from build123d import *

# Parameters (mm, degrees)
BOSS_EXTRUDE1_DEPTH = 8
CUT_EXTRUDE1_DEPTH  = 90
SKETCH3_R           = 5
CUT_EXTRUDE2_DEPTH  = 5.4
SKETCH5_R           = 2.2
SKETCH5_R_2         = 4.65
CUT_EXTRUDE3_DEPTH  = 20
SKETCH6_R           = 20.6
SKETCH6_R_2         = 15.6
CUT_EXTRUDE4_DEPTH  = 2.5
SKETCH7_R           = 20.6
SKETCH7_R_2         = 15.6
CUT_EXTRUDE5_DEPTH  = 2.5
CUT_EXTRUDE6_REACH  = 127.974
SKETCH9_R           = 2.2
SKETCH9_R_2         = 6.575


with BuildPart() as part:
    # Sketch1 → Boss-Extrude1 (new body)
    with BuildSketch(Plane.XY):
        with BuildLine():
            Line((-83.790627288, -89.5), (83.790627288, -89.5))
            ThreePointArc((83.790627288, -89.5), (86.972607803, -88.181980515), (88.290627288, -85))
            Line((88.290627288, -85), (88.290627288, 85))
            ThreePointArc((88.290627288, 85), (86.972607803, 88.181980515), (83.790627288, 89.5))
            Line((83.790627288, 89.5), (-83.790627288, 89.5))
            ThreePointArc((-83.790627288, 89.5), (-86.972607803, 88.181980515), (-88.290627288, 85))
            Line((-88.290627288, 85), (-88.290627288, -85))
            ThreePointArc((-88.290627288, -85), (-86.972607803, -88.181980515), (-83.790627288, -89.5))
        make_face()
    extrude(amount=BOSS_EXTRUDE1_DEPTH)

    # Sketch2 → Cut-Extrude1 (cut)
    with BuildSketch(Plane.XY.offset(8)):
        with BuildLine():
            ThreePointArc((43.745313644, 83.5), (41.145313644, 86.1), (38.545313644, 83.5))
            ThreePointArc((38.545313644, 83.5), (41.145313644, 80.9), (43.745313644, 83.5))
        make_face()
        with BuildLine():
            Line((0, 84), (2.551470164, 84))
            ThreePointArc((2.551470164, 84), (0, 86.1), (-2.551470164, 84))
            Line((-2.551470164, 84), (0, 84))
        make_face()
        with BuildLine():
            Line((0, 84), (-2.551470164, 84))
            ThreePointArc((-2.551470164, 84), (0, 80.9), (2.551470164, 84))
            Line((2.551470164, 84), (0, 84))
        make_face()
        with BuildLine():
            ThreePointArc((-43.745313644, 83.5), (-41.145313644, 80.9), (-38.545313644, 83.5))
            ThreePointArc((-38.545313644, 83.5), (-41.145313644, 86.1), (-43.745313644, 83.5))
        make_face()
        with BuildLine():
            ThreePointArc((-84.890627288, 83.5), (-82.290627288, 80.9), (-79.690627288, 83.5))
            ThreePointArc((-79.690627288, 83.5), (-82.290627288, 86.1), (-84.890627288, 83.5))
        make_face()
        with BuildLine():
            ThreePointArc((-84.890627288, 41.75), (-82.290627288, 39.15), (-79.690627288, 41.75))
            ThreePointArc((-79.690627288, 41.75), (-82.290627288, 44.35), (-84.890627288, 41.75))
        make_face()
        with BuildLine():
            ThreePointArc((-84.890627288, 0), (-82.290627288, -2.6), (-79.690627288, 0))
            ThreePointArc((-79.690627288, 0), (-82.290627288, 2.6), (-84.890627288, 0))
        make_face()
        with BuildLine():
            ThreePointArc((-79.690627288, -83.5), (-82.290627288, -80.9), (-84.890627288, -83.5))
            ThreePointArc((-84.890627288, -83.5), (-82.290627288, -86.1), (-79.690627288, -83.5))
        make_face()
        with BuildLine():
            ThreePointArc((-84.890627288, -41.75), (-82.290627288, -44.35), (-79.690627288, -41.75))
            ThreePointArc((-79.690627288, -41.75), (-82.290627288, -39.15), (-84.890627288, -41.75))
        make_face()
        with BuildLine():
            ThreePointArc((-43.745313644, -83.5), (-41.145313644, -86.1), (-38.545313644, -83.5))
            ThreePointArc((-38.545313644, -83.5), (-41.145313644, -80.9), (-43.745313644, -83.5))
        make_face()
        with BuildLine():
            ThreePointArc((-2.6, -83.5), (0, -86.1), (2.6, -83.5))
            ThreePointArc((2.6, -83.5), (0, -80.9), (-2.6, -83.5))
        make_face()
        with BuildLine():
            ThreePointArc((38.545313644, -83.5), (41.145313644, -86.1), (43.745313644, -83.5))
            ThreePointArc((43.745313644, -83.5), (41.145313644, -80.9), (38.545313644, -83.5))
        make_face()
        with BuildLine():
            ThreePointArc((79.690627288, -83.5), (82.290627288, -86.1), (84.890627288, -83.5))
            ThreePointArc((84.890627288, -83.5), (82.290627288, -80.9), (79.690627288, -83.5))
        make_face()
        with BuildLine():
            ThreePointArc((79.690627288, -41.75), (82.290627288, -44.35), (84.890627288, -41.75))
            ThreePointArc((84.890627288, -41.75), (82.290627288, -39.15), (79.690627288, -41.75))
        make_face()
        with BuildLine():
            ThreePointArc((79.690627288, 0), (82.290627288, -2.6), (84.890627288, 0))
            ThreePointArc((84.890627288, 0), (82.290627288, 2.6), (79.690627288, 0))
        make_face()
        with BuildLine():
            ThreePointArc((79.690627288, 41.75), (82.290627288, 39.15), (84.890627288, 41.75))
            ThreePointArc((84.890627288, 41.75), (82.290627288, 44.35), (79.690627288, 41.75))
        make_face()
        with BuildLine():
            ThreePointArc((79.690627288, 83.5), (82.290627288, 80.9), (84.890627288, 83.5))
            ThreePointArc((84.890627288, 83.5), (82.290627288, 86.1), (79.690627288, 83.5))
        make_face()
    extrude(amount=-CUT_EXTRUDE1_DEPTH, mode=Mode.SUBTRACT)

    # Sketch3 → Cut-Extrude2 (cut)
    with BuildSketch(Plane.XY.offset(8)):
        with Locations((41.145313644, 83.5)):
            Circle(SKETCH3_R)
        with Locations((82.290627288, 83.5)):
            Circle(SKETCH3_R)
        with Locations((82.290627288, 41.75)):
            Circle(SKETCH3_R)
        with Locations((82.290627288, 0)):
            Circle(SKETCH3_R)
        with Locations((82.290627288, -41.75)):
            Circle(SKETCH3_R)
        with Locations((82.290627288, -83.5)):
            Circle(SKETCH3_R)
        with Locations((41.145313644, -83.5)):
            Circle(SKETCH3_R)
        with Locations((0, -83.5)):
            Circle(SKETCH3_R)
        with Locations((-82.290627288, 0)):
            Circle(SKETCH3_R)
        with Locations((-82.290627288, -83.5)):
            Circle(SKETCH3_R)
        with Locations((-82.290627288, -41.75)):
            Circle(SKETCH3_R)
        with Locations((-41.145313644, -83.5)):
            Circle(SKETCH3_R)
        with Locations((-82.290627288, 41.75)):
            Circle(SKETCH3_R)
        with Locations((-82.290627288, 83.5)):
            Circle(SKETCH3_R)
        with Locations((-41.145313644, 83.5)):
            Circle(SKETCH3_R)
        with Locations((0, 83.5)):
            Circle(SKETCH3_R)
    extrude(amount=-CUT_EXTRUDE2_DEPTH, mode=Mode.SUBTRACT)

    # Sketch5 → Cut-Extrude3 (cut)
    with BuildSketch(Plane.XY.offset(8)):
        with Locations((33.49662103, -6.254772237)):
            Circle(SKETCH5_R)
        with Locations((5.99662103, -33.754772237)):
            Circle(SKETCH5_R)
        with Locations((33.49662103, -61.254772237)):
            Circle(SKETCH5_R)
        with Locations((60.99662103, -33.754772237)):
            Circle(SKETCH5_R)
        with Locations((33.49662103, -33.754772237)):
            Circle(SKETCH5_R_2)
    extrude(amount=-CUT_EXTRUDE3_DEPTH, mode=Mode.SUBTRACT)

    # Sketch6 → Cut-Extrude4 (cut)
    with BuildSketch(Plane.XY.offset(8)):
        with Locations((33.49662103, -33.754772237)):
            Circle(SKETCH6_R)
        with Locations((33.49662103, -33.754772237)):
            Circle(SKETCH6_R_2, mode=Mode.SUBTRACT)
    extrude(amount=-CUT_EXTRUDE4_DEPTH, mode=Mode.SUBTRACT)

    # Sketch7 → Cut-Extrude5 (cut)
    with BuildSketch(Plane.XY.offset(8)):
        with Locations((-32.990627288, -34.2)):
            Circle(SKETCH7_R)
        with Locations((-32.990627288, -34.2)):
            Circle(SKETCH7_R_2, mode=Mode.SUBTRACT)
    extrude(amount=-CUT_EXTRUDE5_DEPTH, mode=Mode.SUBTRACT)

    # Sketch9 → Cut-Extrude6 (cut, up to next)
    with BuildSketch(Plane.XY.offset(8), mode=Mode.PRIVATE) as cut_extrude6_sk1:
        with Locations((-5.490627288, -33.754772237)):
            Circle(SKETCH9_R)
    cut_extrude6_tool1 = extrude(cut_extrude6_sk1.sketch, amount=-CUT_EXTRUDE6_REACH, mode=Mode.PRIVATE) & part.part
    # Sketch9 → Cut-Extrude6 (cut, up to next)
    with BuildSketch(Plane.XY.offset(8), mode=Mode.PRIVATE) as cut_extrude6_sk2:
        with Locations((-32.990627288, -6.254772237)):
            Circle(SKETCH9_R)
    cut_extrude6_tool2 = extrude(cut_extrude6_sk2.sketch, amount=-CUT_EXTRUDE6_REACH, mode=Mode.PRIVATE) & part.part
    # Sketch9 → Cut-Extrude6 (cut, up to next)
    with BuildSketch(Plane.XY.offset(8), mode=Mode.PRIVATE) as cut_extrude6_sk3:
        with Locations((-32.990627288, -61.254772237)):
            Circle(SKETCH9_R)
    cut_extrude6_tool3 = extrude(cut_extrude6_sk3.sketch, amount=-CUT_EXTRUDE6_REACH, mode=Mode.PRIVATE) & part.part
    # Sketch9 → Cut-Extrude6 (cut, up to next)
    with BuildSketch(Plane.XY.offset(8), mode=Mode.PRIVATE) as cut_extrude6_sk4:
        with Locations((-32.990627288, -34.2)):
            Circle(SKETCH9_R_2)
    cut_extrude6_tool4 = extrude(cut_extrude6_sk4.sketch, amount=-CUT_EXTRUDE6_REACH, mode=Mode.PRIVATE) & part.part
    # Sketch9 → Cut-Extrude6 (cut, up to next)
    with BuildSketch(Plane.XY.offset(8), mode=Mode.PRIVATE) as cut_extrude6_sk5:
        with Locations((-60.490627288, -33.754772237)):
            Circle(SKETCH9_R)
    cut_extrude6_tool5 = extrude(cut_extrude6_sk5.sketch, amount=-CUT_EXTRUDE6_REACH, mode=Mode.PRIVATE) & part.part
    add(cut_extrude6_tool1.solids().sort_by_distance((-5.490627, -33.754772, 8))[0], mode=Mode.SUBTRACT)
    add(cut_extrude6_tool2.solids().sort_by_distance((-32.990627, -6.254772, 8))[0], mode=Mode.SUBTRACT)
    add(cut_extrude6_tool3.solids().sort_by_distance((-32.990627, -61.254772, 8))[0], mode=Mode.SUBTRACT)
    add(cut_extrude6_tool4.solids().sort_by_distance((-32.990627, -34.2, 8))[0], mode=Mode.SUBTRACT)
    add(cut_extrude6_tool5.solids().sort_by_distance((-60.490627, -33.754772, 8))[0], mode=Mode.SUBTRACT)


solid = part.part
Verification items for the finished model (mm, model axes). A direction names the side the tool comes from. Give positions to 0.01 mm unless a question says otherwise; leave off trailing zeros. Loops run counter-clockwise (first coordinate to the right, second up) from the corner with the lowest first, then second, coordinate; pieces in that order, holes last.
1. Cross-section at C-C on x = -20. Record the cut outline in (y, z).
Derived:
outline: (-89.5, 0) - (89.5, 0) - (89.5, 8) - (-18.21, 8) - (-18.21, 5.5) - (-25.56, 5.5) - (-25.56, 8) - (-42.84, 8) - (-42.84, 5.5) - (-50.19, 5.5) - (-50.19, 8) - (-89.5, 8) - close
2. Cross-section at A-A on y = 41.75. Record the cut outline in (x, z).
Derived:
outline: (-88.29, 0) - (-84.89, 0) - (-84.89, 2.6) - (-87.29, 2.6) - (-87.29, 8) - (-88.29, 8) - close; (-79.69, 0) - (79.69, 0) - (79.69, 2.6) - (77.29, 2.6) - (77.29, 8) - (-77.29, 8) - (-77.29, 2.6) - (-79.69, 2.6) - close; (84.89, 0) - (88.29, 0) - (88.29, 8) - (87.29, 8) - (87.29, 2.6) - (84.89, 2.6) - close
3. Material ranges on probe 1 along X at (y, z) = (0, 0.8); probe 2 along Y at (x, z) = (0, 0.7); probe 3 along Y at (x, z) = (81.5, 1.5), recorded low to high.
Derived:
probe 1: x = -88.29 to -84.89, -79.69 to 79.69, 84.89 to 88.29
probe 2: y = -89.5 to -86.1, -80.9 to 80.9, 86.1 to 89.5
probe 3: y = -89.5 to -85.98, -81.02 to -44.23, -39.27 to -2.48, 2.48 to 39.27, 44.23 to 81.02, 85.98 to 89.5
4. Tool access check on faces 1 (the flat face through (84, 81, 2.6)), 2 (the cylindrical face through (86.937, -88.217, 3.944)). Record the directions out of +Z, -Z, +X, -X, +Y, -Y that give a thin tool (end or side, any length) a straight path to the whole face; none if there is none.
Derived:
face 1: +Z
face 2: +Z, -Z, +X, -Y
5. Cross-section at B-B on z = 4. Count the separate pieces of the cut face and the enclosed holes in it, and give its area (3 significant figures).
Derived:
separate pieces: 1
enclosed holes: 26
area: 30,000 mm2
6. Go/stop test with flat-tipped pins: P1, Ø4, axis at x = 41.15, y = 83.5, coming from the +Z side; P2, Ø5, axis at x = -81.5, y = -42.5, coming from the +Z side; P3, Ø5, axis at x = -33, y = -28.5, coming from the +Z side. Record where each tip stops, or that it passes through.
Derived:
P1: passes through
P2: stops at z = 2.6
P3: stops at z = 8
